Input: part model. Units: mm. Frame: model coordinates. Give positions to 0.01 mm unless a question says otherwise; leave off trailing zeros. Loops run counter-clockwise (first coordinate to the right, second up) from the corner with the lowest first, then second, coordinate; pieces in that order, holes last.
Autodesk Inventor part; units mm, degrees
ref_plane "YZ Plane" through (0, 0, 0) normal (1, 0, 0) x (0, 1, 0)
ref_plane "XY Plane" through (0, 0, 0) normal (0, 0, 1) x (1, 0, 0)
sketch "Skizze1" plane through (0, 0, 0) normal (0, 0, 1) x (1, 0, 0)
  line L0 (0, 0) -> (5, 0)
  line L1 (5, 0) -> (5, 8)
  line L2 (5, 8) -> (4, 8)
  line L3 (4, 8) -> (4, 1)
  line L4 (4, 1) -> (0, 1)
  line L5 (0, 9.6) -> (0, -1.6) construction
  line L6 (0, 0) -> (-5, 0)
  line L7 (-5, 0) -> (-5, 8)
  line L8 (-5, 8) -> (-4, 8)
  line L9 (-4, 8) -> (-4, 1)
  line L10 (-4, 1) -> (0, 1)
  dimension "d0" = 1
  dimension "d1" = 1
  dimension "d2" = 8
  dimension "d3" = 5
extrude "Ex-UProfil" add sketch "Skizze1" along normal blind 660
sketch "Skizze2" plane through (0, 0, 0) normal (0, 1, 0) x (-1, 0, 0)
  line L0 (5, 0) -> (-5, 0)
  line L1 (-5, 0) -> (-5, 660)
  line L2 (5, 660) -> (-5, 660)
  line L3 (5, 0) -> (5, 660)
  line L4 (0, -53) -> (0, 318) construction
  circle A0 centre (0, 650) radius 2.15 construction
  line L5 (0, 651) -> (0, 649) construction
  line L6 (-2.15, 651) -> (-2.15, 649)
  line L7 (2.15, 649) -> (2.15, 651)
  arc A1 (2.15, 651) -> (-2.15, 651) centre (0, 651) ccw
  arc A2 (-2.15, 649) -> (2.15, 649) centre (0, 649) ccw
  circle A3 centre (0, 570) radius 2.15 construction
  line L8 (0, 571) -> (0, 569) construction
  line L9 (-2.15, 571) -> (-2.15, 569)
  line L10 (2.15, 569) -> (2.15, 571)
  arc A4 (2.15, 571) -> (-2.15, 571) centre (0, 571) ccw
  arc A5 (-2.15, 569) -> (2.15, 569) centre (0, 569) ccw
  circle A6 centre (0, 490) radius 2.15 construction
  line L11 (0, 491) -> (0, 489) construction
  line L12 (-2.15, 491) -> (-2.15, 489)
  line L13 (2.15, 489) -> (2.15, 491)
  arc A7 (2.15, 491) -> (-2.15, 491) centre (0, 491) ccw
  arc A8 (-2.15, 489) -> (2.15, 489) centre (0, 489) ccw
  circle A9 centre (0, 410) radius 2.15 construction
  line L14 (0, 411) -> (0, 409) construction
  line L15 (-2.15, 411) -> (-2.15, 409)
  line L16 (2.15, 409) -> (2.15, 411)
  arc A10 (2.15, 411) -> (-2.15, 411) centre (0, 411) ccw
  arc A11 (-2.15, 409) -> (2.15, 409) centre (0, 409) ccw
  circle A12 centre (0, 330) radius 2.15 construction
  line L17 (0, 331) -> (0, 329) construction
  line L18 (-2.15, 331) -> (-2.15, 329)
  line L19 (2.15, 329) -> (2.15, 331)
  arc A13 (2.15, 331) -> (-2.15, 331) centre (0, 331) ccw
  arc A14 (-2.15, 329) -> (2.15, 329) centre (0, 329) ccw
  circle A15 centre (0, 250) radius 2.15 construction
  line L20 (0, 251) -> (0, 249) construction
  line L21 (-2.15, 251) -> (-2.15, 249)
  line L22 (2.15, 249) -> (2.15, 251)
  arc A16 (2.15, 251) -> (-2.15, 251) centre (0, 251) ccw
  arc A17 (-2.15, 249) -> (2.15, 249) centre (0, 249) ccw
  circle A18 centre (0, 170) radius 2.15 construction
  line L23 (0, 171) -> (0, 169) construction
  line L24 (-2.15, 171) -> (-2.15, 169)
  line L25 (2.15, 169) -> (2.15, 171)
  arc A19 (2.15, 171) -> (-2.15, 171) centre (0, 171) ccw
  arc A20 (-2.15, 169) -> (2.15, 169) centre (0, 169) ccw
  circle A21 centre (0, 90) radius 2.15 construction
  line L26 (0, 91) -> (0, 89) construction
  line L27 (-2.15, 91) -> (-2.15, 89)
  line L28 (2.15, 89) -> (2.15, 91)
  arc A22 (2.15, 91) -> (-2.15, 91) centre (0, 91) ccw
  arc A23 (-2.15, 89) -> (2.15, 89) centre (0, 89) ccw
  circle A24 centre (0, 10) radius 2.15 construction
  line L29 (0, 11) -> (0, 9) construction
  line L30 (-2.15, 11) -> (-2.15, 9)
  line L31 (2.15, 9) -> (2.15, 11)
  arc A25 (2.15, 11) -> (-2.15, 11) centre (0, 11) ccw
  arc A26 (-2.15, 9) -> (2.15, 9) centre (0, 9) ccw
  point P0 (0, 0)
  point P1 (0, 653.15)
  point P2 (0, 646.85)
  point P3 (0, 573.15)
  point P4 (0, 566.85)
  point P5 (0, 493.15)
  point P6 (0, 486.85)
  point P7 (0, 413.15)
  point P8 (0, 406.85)
  point P9 (0, 333.15)
  point P10 (0, 326.85)
  point P11 (0, 253.15)
  point P12 (0, 246.85)
  point P13 (0, 173.15)
  point P14 (0, 166.85)
  point P15 (0, 93.15)
  point P16 (0, 86.85)
  point P17 (0, 13.15)
  point P18 (0, 6.85)
  dimension "d6" = 4.3
  dimension "d7" = 10
  dimension "d8" = 4.3
  dimension "d9" = 6.3
  dimension "d21" = 80
extrude "Ex-Bohrungen" cut sketch "Skizze2" along normal up to surface (1 mm away) contours A1 L7 A2 L6 | A4 L10 A5 L9 | A7 L13 A8 L12 | A10 L16 A11 L15 | A13 L19 A14 L18 | A16 L22 A17 L21 | A19 L25 A20 L24 | A22 L28 A23 L27 | A25 L31 A26 L30
equation "\"d8\" = d6"
properties part number "U-Profil PanelSupport 10x8x660mm"
(1) Cut plane C-C (x = 0). Count the separate pieces of the cut face and the enclosed holes in it, and give its area (3 significant figures).
Values follow:
separate pieces: 10
enclosed holes: 0
area: 603 mm2
(2) Ray query, probe 1 along X at (y, z) = (2.5, 452); probe 2 along Y at (x, z) = (-2.25, 219). Return the intervals inside material, ascending.
Values follow:
probe 1: x = -5 to -4, 4 to 5
probe 2: y = 0 to 1
(3) Cut plane A-A (y = 6.5). Return the cut outline in (x, z), and give its area (3 significant figures).
Values follow:
outline: (-5, 0) - (-4, 0) - (-4, 660) - (-5, 660) - close; (4, 0) - (5, 0) - (5, 660) - (4, 660) - close
area: 1,320 mm2
(4) Cut plane B-B (z = 521.5). Return the cut outline in (x, y).
Values follow:
outline: (-5, 0) - (5, 0) - (5, 8) - (4, 8) - (4, 1) - (-4, 1) - (-4, 8) - (-5, 8) - close
(5) Pin query (flat end, axial travel): pin 1 Ø4 at (x, y) = (3, 2) entering from +Z; pin 2 Ø3 at (x, z) = (1.5, 478) entering from +Y. Return the tip coordinate at first contact, or that it passes through.
Values follow:
pin 1: stops at z = 660
pin 2: stops at y = 1
